from build123d import *

# Parameters (mm, degrees)
SKETCH_1_W          = 27.7
SKETCH_1_H          = 15.8
EXTRUDE_1_DEPTH     = 5
SKETCH_2_R          = 1.3
CUT_EXTRUDE_1_DEPTH = 17.710251345
SKETCH_3_R          = 1.3
EXTRUDE_2_DEPTH     = 5
FILLET_1_R          = 3


with BuildPart() as part:
    # ｽｹｯﾁ1 → ﾎﾞｽ - 押し出し1 (new body)
    with BuildSketch(Plane(origin=(0, 0, 0), x_dir=(1, 0, 0), z_dir=(0, 1, 0))):
        Rectangle(SKETCH_1_W, SKETCH_1_H)
    extrude(amount=EXTRUDE_1_DEPTH)

    # ｽｹｯﾁ2 → ｶｯﾄ - 押し出し1 (cut, through all)
    with BuildSketch(Plane(origin=(0, 5, 0), x_dir=(1, 0, 0), z_dir=(0, 1, 0))):
        with Locations(Location((-11.25, 5.3, 0), (0, 0, 270))):
            Circle(SKETCH_2_R)
        with Locations(Location((11.25, -5.3, 0), (0, 0, 270))):
            Circle(SKETCH_2_R)
    extrude(amount=-CUT_EXTRUDE_1_DEPTH, mode=Mode.SUBTRACT)

    # ｽｹｯﾁ3 → ﾎﾞｽ - 押し出し2 (add)
    # profile 1 of 2: a face of its own
    with BuildSketch(Plane(origin=(0, 5, 0), x_dir=(1, 0, 0), z_dir=(0, 1, 0))):
        Polygon((25.37, -6.15), (13.85, -6.15), (13.85, -7.9), (-13.85, -7.9), (-13.85, -16.15), (25.37, -16.15), align=None)
        with Locations(Location((-8.85, -11.15, 0), (0, 0, 270))):
            Circle(SKETCH_3_R, mode=Mode.SUBTRACT)
        with Locations(Location((20.37, -11.15, 0), (0, 0, 270))):
            Circle(SKETCH_3_R, mode=Mode.SUBTRACT)
    # profile 2 of 2: a face of its own
    with BuildSketch(Plane(origin=(0, 5, 0), x_dir=(1, 0, 0), z_dir=(0, 1, 0))):
        Polygon((13.85, 7.9), (13.85, -6.15), (25.37, -6.15), align=None)
    extrude(amount=-EXTRUDE_2_DEPTH)

    # ﾌｨﾚｯﾄ1
    fillet_1_edges = [part.edges().sort_by_distance(p)[0] for p in [
        (-13.85, 2.5, 16.15),
        (25.37, 2.5, 16.15),
        (25.37, 2.5, 6.15),
        (-13.85, 2.5, -7.9),
        (13.85, 2.5, -7.9),
    ]]
    fillet(fillet_1_edges, radius=FILLET_1_R)


solid = part.part
Can you work these out from the model? Positions are in its coordinate system, mm. Coordinates: 2 decimals unless noted, no trailing zeros. Write each loop counter-clockwise with the first axis right and the second up, starting at its lowest first coordinate (ties: lowest second). Pieces come first, ordered by that corner, then holes.
Q1. Imagine slicing it at B-B, the plane y = 0.8. List the corners of the cut face in (x, z) for me, plus the area to 3 significant figures.
Results found:
outline: (-13.85, -4.9) arc R3 ccw to (-10.85, -7.9) - (12.43, -7.9) arc R3 ccw to (14.75, -6.8) - (24.69, 5.32) arc R3 ccw to (25.37, 7.22) - (25.37, 13.15) arc R3 ccw to (22.37, 16.15) - (-10.85, 16.15) arc R3 ccw to (-13.85, 13.15) - close; hole circle Ø2.6 at (-11.25, -5.3); hole circle Ø2.6 at (-8.85, 11.15); hole circle Ø2.6 at (11.25, 5.3); hole circle Ø2.6 at (20.37, 11.15)
area: 835 mm2
Q2. Imagine slicing it at D-D, the plane x = 20.37. List the corners of the cut face in (y, z) for me, plus the area to 3 significant figures.
Results found:
outline: (0, 0.05) - (5, 0.05) - (5, 9.85) - (0, 9.85) - close; (0, 12.45) - (5, 12.45) - (5, 16.15) - (0, 16.15) - close
area: 67.5 mm2
Q3. Imagine slicing it at C-C, the plane z = 10.5. List the corners of the cut face in (x, y) for me, plus the area to 3 significant figures.
Results found:
outline: (-13.85, 0) - (-9.98, 0) - (-9.98, 5) - (-13.85, 5) - close; (-7.72, 0) - (19.24, 0) - (19.24, 5) - (-7.72, 5) - close; (21.5, 0) - (25.37, 0) - (25.37, 5) - (21.5, 5) - close
area: 174 mm2
Q4. If we mould it in two halves opening along Z, with no side actions, what happens to faces 1 (the face through (12.54, 2.54, 5.13)), 2 (the face through (24.51, 2.46, 15.25)), 3 (the face through (13.7, 2.54, -7.62))? For each: +Z half, -Z half, draft (parallel to the pull), parting line (faces both ways), or undercut.
Results found:
face 1: undercut
face 2: +Z half
face 3: -Z half
Q5. Imagine slicing it at A-A, the plane x = -8.85. List the corners of the cut face in (y, z) for me, plus the area to 3 significant figures.
Results found:
outline: (0, -7.9) - (5, -7.9) - (5, 9.85) - (0, 9.85) - close; (0, 12.45) - (5, 12.45) - (5, 16.15) - (0, 16.15) - close
area: 107 mm2
Q6. For P1, Ø1.5, axis at y = 3.5, z = -2.5, coming from the +X side; P2, Ø3, axis at x = 17.5, y = 2, coming from the -Z side, each with a flat end and sliding along its axis, tell me the tip position at first contact or that it passes through.
Results found:
P1: stops at x = 18.89
P2: stops at z = -5.28
Q7. Please list where these lines run through material, in increasing order: L1, parallel to X at y = 3.2, z = 11.15; L2, parallel to X at y = 2.2, z = -5.3; L3, parallel to X at y = 3.85, z = 5.3.
Results found:
L1: x = -13.85 to -10.15, -7.55 to 19.07, 21.67 to 25.37
L2: x = -13.82 to -12.55, -9.95 to 15.98
L3: x = -13.85 to 9.95, 12.55 to 24.67
